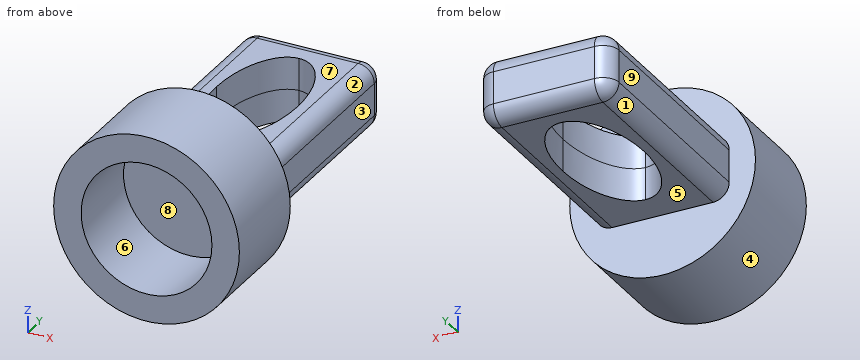
Autodesk Fusion 360 part; units mm, degrees
sketch "Sketch1" plane through (0, 0, 0) normal (0, 1, 0) x (1, 0, 0)
  circle A0 centre (0, 0) radius 8.1
  circle A1 centre (0, 0) radius 11.5
  dimension "d1" = 16.2
  dimension "d2" = 23
extrude "Extrude1" add sketch "Sketch1" along normal blind 10
extrude "Extrude2" add sketch "Sketch1" along normal blind 2 from surface at 10 contours A0 | A1
sketch "Sketch2" plane through (0, 0, 0) normal (0, 0, 1) x (1, 0, 0)
  ellipse E0 centre (0, 26) end of major axis (0, 36) minor radius 5
  line L0 (0, 16) -> (0, 36)
  line L1 (5, 26) -> (-5, 26)
  dimension "d8" = 20
  dimension "d9" = 10
  dimension "d10" = 26
sketch "Sketch3" plane through (0, 0, 0) normal (0, 0, 1) x (1, 0, 0)
  line L0 (8.25, 12) -> (-8.25, 12)
  line L1 (-8.25, 12) -> (-8.25, 40)
  line L2 (-8.25, 40) -> (8.25, 40)
  line L3 (8.25, 40) -> (8.25, 12)
  line L4 (8.25, 12) -> (-8.25, 40) construction
  line L5 (-8.25, 12) -> (8.25, 40) construction
  point P0 (0, 26)
  dimension "d11" = 16.5
  dimension "d12" = 28
  dimension "d13" = 12
extrude "Extrude3" add sketch "Sketch3" along normal mid plane 8
extrude "Extrude4" cut sketch "Sketch2" along normal mid plane 20
fillet "Fillet1" radius 2 8 edges at (8.25, 26, 4) (8.25, 26, -4) (0, 40, 4) (0, 40, -4) (8.25, 40, 0) (-8.25, 40, 0) (-8.25, 26, 4) (-8.25, 26, -4)
Design review of the part built by this model. Coordinates are the model's own, in mm. Face numbers are marked on the shaded views. A direction names the side the tool comes from. Coordinates: 2 decimals unless noted, no trailing zeros. Loops run counter-clockwise (first coordinate to the right, second up) from the corner with the lowest first, then second, coordinate; pieces in that order, holes last.
Item 1: Wall thickness on L1, parallel to Z at x = 0, y = 3; L2, parallel to X at y = 7, z = -1.25: over which ranges is each line inside the solid? List them lowest first.
Completed:
L1: z = -11.5 to -8.1, 8.1 to 11.5
L2: x = -11.43 to -8, 8 to 11.43
Item 2: Add section C-C (y = 3). Write out the cut boundary in (x, z).
Completed:
outline: circle Ø23 at (0, 0); hole circle Ø16.2 at (0, 0)
Item 3: Add section A-A (y = 15). Write out the cut boundary in (x, z), and give its area (3 significant figures).
Completed:
outline: (-8.25, -2) arc R2 ccw to (-6.25, -4) - (6.25, -4) arc R2 ccw to (8.25, -2) - (8.25, 2) arc R2 ccw to (6.25, 4) - (-6.25, 4) arc R2 ccw to (-8.25, 2) - close
area: 129 mm2
Item 4: Add section B-B (z = -4.5). Write out the cut boundary in (x, y).
Completed:
outline: (-10.58, 0) - (-6.73, 0) - (-6.73, 10) - (6.73, 10) - (6.73, 0) - (10.58, 0) - (10.58, 12) - (-10.58, 12) - close
Item 5: For the marked faces 1, 2, 3, 4 and 5, list the 3-axis set-ups (+Z, -Z, +X, -X, +Y, -Y) from which the entire face can be reached by the end or side of a thin tool; tool diameter is ignored.
Completed:
face 1: -Z, -X, +Y
face 2: +Z, +X, +Y
face 3: +Z, -Z, +X, +Y
face 4: +Y, -Y
face 5: -Z, +X, -X, +Y
Item 6: Add section D-D (x = -7). Write out the cut boundary in (y, z), and give its area (3 significant figures).
Completed:
outline: (0, -9.12) - (12, -9.12) - (12, -3.85) - (38, -3.85) arc R1.85 ccw to (39.85, -2) - (39.85, 2) arc R1.85 ccw to (38, 3.85) - (12, 3.85) - (12, 9.12) - (0, 9.12) - (0, 4.08) - (10, 4.08) - (10, -4.08) - (0, -4.08) - close
area: 351 mm2
Item 7: Draft analysis for pull direction Z (two halves, no side actions). For the marked faces 6, 7, 8 and 9, state which applies: pulls with the +Z half, pulls with the -Z half, needs draft (parallel to the pull), parting line crosses it, or undercut.
Completed:
face 6: undercut
face 7: pulls with the +Z half
face 8: undercut
face 9: needs draft
Item 8: Clearance check with flat-ended pins moving along their axes: pin 1 (5 mm diameter, centred on x = 0, z = 1.5, fed in from -Y); pin 2 (8 mm diameter, centred on y = 22, z = -3.5, fed in from +X); pin 3 (3 mm diameter, centred on y = 27, z = -0.5, fed in from -X); pin 4 (6.5 mm diameter, centred on x = -0.5, y = 27, fed in from -Z). State where each tip first meets the part, or that it passes through.
Completed:
pin 1: stops at y = 10
pin 2: stops at x = 8.25
pin 3: stops at x = -8.25
pin 4: passes through
